```python
from build123d import *

# Parameters (mm, degrees)
F0_R     = 6.1031552094
F2_DEPTH = 6
F3_R     = 3
F4_DEPTH = 3
F5_R     = 5
F6_R     = 2


with BuildPart() as f2:
    # F0 (on Front) → F2 (new body)
    with BuildSketch(Plane.XZ):
        Circle(F0_R)
    extrude(amount=F2_DEPTH)

    # F3
    f3_edges = [f2.edges().sort_by_distance(p)[0] for p in [
        (-6.103155, -6, 0),
    ]]
    fillet(f3_edges, radius=F3_R)

    # F1 (on Front) → F4 (join)
    with BuildSketch(Plane.XZ):
        Polygon((-3.1815413386, -5.0610057078), (3.1815413386, -5.0610057078), (24.3407674134, -14.5224481821), (24.3407674134, 14.5224481821), (3.1815413386, 5.0610057078), (-3.1815413386, 5.0610057078), (-24.3407674134, 14.5224481821), (-24.3407674134, -14.5224481821), align=None)
    extrude(amount=F4_DEPTH)

    # F5
    f5_edges = [f2.edges().sort_by_distance(p)[0] for p in [
        (24.340767, -1.5, 14.522448),
        (24.340767, -1.5, -14.522448),
        (-24.340767, -1.5, -14.522448),
        (-24.340767, -1.5, 14.522448),
    ]]
    fillet(f5_edges, radius=F5_R)

    # F6
    f6_edges = [f2.edges().sort_by_distance(p)[0] for p in [
        (-22.060594, -3, -11.005109),
        (10.309065, -3, 8.24811),
    ]]
    fillet(f6_edges, radius=F6_R)


solid = f2.part
```
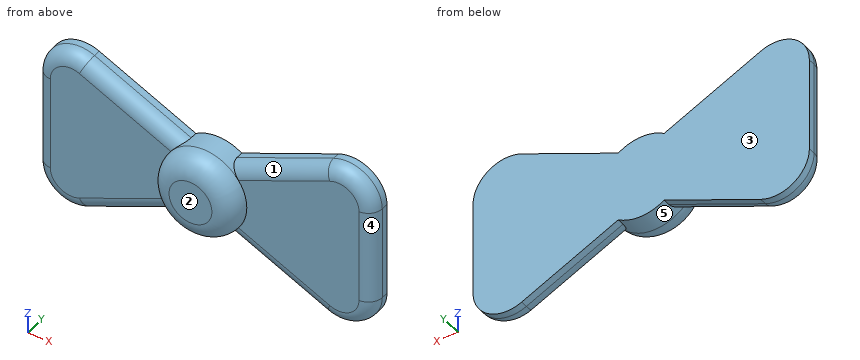
For this review, take the finished solid that the model builds, in its own axes (mm). Face numbers are marked on the shaded views. A direction names the side the tool comes from. Give positions to 0.01 mm unless a question says otherwise; leave off trailing zeros. Write each loop counter-clockwise with the first axis right and the second up, starting at its lowest first coordinate (ties: lowest second). Pieces come first, ordered by that corner, then holes. Notation, with made-up numbers: M -25,11.5 L -11,11.5 A33 ccw -11,47.5 Z; hole C 15.5,-38.5 d10. An arc over 180 degrees is marked long. Answer as CSV lines item,"result".
1. Consider section B-B, the plane y = -2.5. Write out the cut boundary in (x, z), then the cut area to 3 significant figures.
Findings:
outline,"M -23.66,-6.81 A4.32 ccw -17.58,-10.76 L -3.94,-4.66 A6.1 ccw 3.94,-4.66 L 17.58,-10.76 A4.32 ccw 23.66,-6.81 L 23.66,6.81 A4.32 ccw 17.58,10.76 L 3.94,4.66 A6.1 ccw -3.94,4.66 L -17.58,10.76 A4.32 ccw -23.66,6.81 Z"
area,"764 mm2"
2. Consider section A-A, the plane y = -0.5. Write out the cut boundary in (x, z).
Findings:
outline,"M -24.34,-6.81 A5 ccw -17.3,-11.37 L -3.32,-5.12 A6.1 ccw 3.32,-5.12 L 17.3,-11.37 A5 ccw 24.34,-6.81 L 24.34,6.81 A5 ccw 17.3,11.37 L 3.32,5.12 A6.1 ccw -3.32,5.12 L -17.3,11.37 A5 ccw -24.34,6.81 Z"
3. Wall thickness on line 1 (Y direction, x = 17, z = -1.25); line 2 (X direction, y = -1.75, z = 10.5); line 3 (X direction, y = -1.5, z = 8.75): over which ranges is each line inside the solid? List them lowest first.
Findings:
line 1,"y = -3 to 0"
line 2,"x = -22.49 to -15.7, 15.7 to 22.49"
line 3,"x = -23.88 to -11.59, 11.59 to 23.88"
4. Draft analysis for pull direction X (two halves, no side actions). For the marked faces 3, 4 and 5, state which applies: +X half, -X half, draft (parallel to the pull), parting line (faces both ways), or undercut.
Findings:
face 3,"draft"
face 4,"+X half"
face 5,"undercut"
5. Consider section C-C, the plane y = -4.75. Write out the cut boundary in (x, z), then the cut area to 3 significant figures.
Findings:
outline,"C 0,0 d11.08"
area,"96.4 mm2"
6. For the marked faces 1 and 2, list the 3-axis set-ups (+Z, -Z, +X, -X, +Y, -Y) from which the entire face can be reached by the end or side of a thin tool; tool diameter is ignored.
Findings:
face 1,"+Z, -Y"
face 2,"+Z, -Z, +X, -X, -Y"
7. For pin 1 (1.5 mm diameter, centred on x = 14, y = -1.5, fed in from +Z); pin 2 (3 mm diameter, centred on x = -14, z = 0.5, fed in from -Y); pin 3 (3 mm diameter, centred on x = 18.5, y = -2.5, fed in from -Z), all flat-tipped, find the tip position at first contact; note any pin that passes through.
Findings:
pin 1,"stops at z = 10.2"
pin 2,"stops at y = -3"
pin 3,"stops at z = -11.8"
